CAD build for the part. Positions are in the model's coordinates, mm. Face numbers are marked on the shaded views. A direction names the side the tool comes from. Give positions to 0.01 mm unless a question says otherwise; leave off trailing zeros. Write each loop counter-clockwise with the first axis right and the second up, starting at its lowest first coordinate (ties: lowest second). Pieces come first, ordered by that corner, then holes. Notation, with made-up numbers: (21.5, 3.5) -> (32.5, 3.5) arc R22 ccw to (32.5, 21.5) -> close; hole circle Ø3 at (-35.5, 19.5). An arc over 180 degrees is marked (long way). Use one line per item in the form item = value. Start each with the question number.
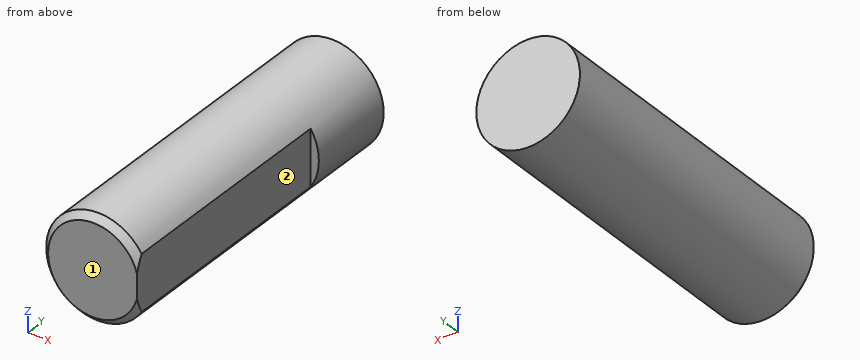
from build123d import *

# Parameters (mm, degrees)
SKETCH015_R          = 3.175
PAD009_DEPTH         = 20.6
SKETCH016_W          = 0.5
SKETCH016_H          = 15
POCKET008_DEPTH      = 3.176
POCKET008_DEPTH_BACK = 3.176
CHAMFER_SIZE         = 0.4


with BuildPart() as part:
    # Sketch015 → Pad009 (new body)
    with BuildSketch(Plane.XZ):
        Circle(SKETCH015_R)
    extrude(amount=PAD009_DEPTH)

    # Sketch016 → Pocket008 (cut, two sides)
    with BuildSketch(Plane.XY) as pocket008_sk:
        with Locations((2.925, -13.1)):
            Rectangle(SKETCH016_W, SKETCH016_H)
    extrude(amount=-POCKET008_DEPTH, mode=Mode.SUBTRACT)
    extrude(pocket008_sk.sketch, amount=POCKET008_DEPTH_BACK, mode=Mode.SUBTRACT)

    # Chamfer
    chamfer_edges = [part.edges().sort_by_distance(p)[0] for p in [
        (-3.175, -20.6, 0),
    ]]
    chamfer(chamfer_edges, length=CHAMFER_SIZE)


solid = part.part
1) Pin check, flat tips, straight feed: pin 1 (2.5 mm diameter, centred on y = -13.5, z = -0.5, fed in from +X) (3 decimals); pin 2 (1 mm diameter, centred on x = 1, y = -17, fed in from -Z); pin 3 (2 mm diameter, centred on y = -14.5, z = -1.5, fed in from -X). Stop position of each tip, or through.
2) Wall check: line 1 along X through (y, z) = (-14.25, 2); line 2 along X through (y, z) = (-18.75, 1.75); line 3 along Z through (x, y) = (1.5, -11.5). Give the ranges that are in metal, low to high. Write a range as from..to.
3) Cut at B-B (y = -15.5). Give the cut face in (x, z) (3 decimals).
4) 3-axis set-ups, long thin cutter, end or side, ignore diameter. For the marked faces 1 and 2: which of +Z, -Z, +X, -X, +Y, -Y reach the whole face in a straight line?
5) Cut at A-A (z = 0). Give the cut face in (x, y) (3 decimals), and give its area (3 significant figures).
Final values:
q1.pin_1 = 2.675
q1.pin_2 = -3.14
q1.pin_3 = -3.14
q2.line_1 = -2.47..2.47
q2.line_2 = -2.65..2.65
q2.line_3 = -2.8..2.8
q3.outline = (2.675, -1.71) -> (2.675, 1.71) arc R3.175 ccw (long way) to start
q4.face_1 = +Z, -Z, +X, -X, -Y
q4.face_2 = +Z, -Z, +X, -Y
q5.outline = (-3.175, -20.2) -> (-2.775, -20.6) -> (2.675, -20.6) -> (2.675, -5.6) -> (3.175, -5.6) -> (3.175, 0) -> (-3.175, 0) -> close
q5.area = 123 mm^2
